Can you work these out from the model? Positions are in its coordinate system, mm. A direction names the side the tool comes from. Give positions to 0.01 mm unless a question says otherwise; leave off trailing zeros. Loops run counter-clockwise (first coordinate to the right, second up) from the corner with the lowest first, then second, coordinate; pieces in that order, holes last. Notation, with made-up numbers: (76.25, -26.5) - (103.25, -26.5) arc R22 cw to (103.25, -5.5) - close; hole circle Ø9 at (78, -14). An arc over 180 degrees is marked (long way). Answer in a Markdown table with one row per item.
from build123d import *

# Parameters (mm, degrees)
SKETCH_1_R      = 7.5
SKETCH_1_R_2    = 4
EXTRUDE_1_DEPTH = 24
SKETCH_4_W      = 1
SKETCH_4_H      = 1
FILLET_1_R      = 0.2


with BuildPart() as part:
    # 草图1 → 凸台-拉伸1 (new body)
    with BuildSketch(Plane.XY):
        Circle(SKETCH_1_R)
        Circle(SKETCH_1_R_2, mode=Mode.SUBTRACT)
    extrude(amount=EXTRUDE_1_DEPTH)

    # 草图4 → 切除-旋转1 (revolve, cut)
    with BuildSketch(Plane(origin=(0, 0, 0), x_dir=(0, 0, -1), z_dir=(1, 0, 0)), mode=Mode.PRIVATE) as cut_revolve_1_sk:
        with Locations((-20.5, 7.016772844)):
            Rectangle(SKETCH_4_W, SKETCH_4_H)
        with Locations((-3.5, 7.016772844)):
            Rectangle(SKETCH_4_W, SKETCH_4_H)
    revolve(cut_revolve_1_sk.sketch.rotate(Axis((0, 0, 0), (0, 0, 1)), 90), axis=Axis((0, 0, 0), (0, 0, 1)), mode=Mode.SUBTRACT)

    # 圆角1
    fillet_1_edges = [part.edges().sort_by_distance(p)[0] for p in [
        (-7.5, 0, 21),
        (-7.5, 0, 20),
        (-7.5, 0, 4),
        (-7.5, 0, 3),
    ]]
    fillet(fillet_1_edges, radius=FILLET_1_R)


solid = part.part
Q1. For pin 1 (5 mm diameter, centred on x = -5, z = 13, fed in from +Y); pin 2 (8 mm diameter, centred on y = 6, z = 8.5, fed in from +X); pin 3 (1.5 mm diameter, centred on x = -1, z = 6.5, fed in from -Y), each with a flat end and sliding along its axis, tell me the tip position at first contact or that it passes through.
Checked values:
| item | result |
|---|---|
| pin 1 | stops at y = 7.07 |
| pin 2 | stops at x = 7.23 |
| pin 3 | stops at y = -7.5 |
Q2. If we mould it in two halves opening along Z, with no side actions, what happens to faces 1 (the face through (1.413, 6.362, 20.493)), 2 (the face through (3, -3, 0)), 3 (the face through (-7.493, 0.33, 22.58))? For each: released by +Z, released by -Z, zero draft, split by the parting line, or undercut.
Checked values:
| item | result |
|---|---|
| face 1 | undercut |
| face 2 | released by -Z |
| face 3 | zero draft |
Q3. On a 3-axis mill with a long thin cutter (end or side, diameter ignored), from which of +Z, -Z, +X, -X, +Y, -Y can I reach the whole of each face in a straight line? I mean faces 4 (the face through (-3, -6, 3)), 5 (the face through (-7.493, 0.33, 1.38)). Say none if no direction works.
Checked values:
| item | result |
|---|---|
| face 4 | none |
| face 5 | +Z, -Z |
Q4. Imagine slicing it at C-C, the plane z = 8.75. Write out the boundary of the cut face in (x, y), and give its area (3 significant figures).
Checked values:
| item | result |
|---|---|
| outline | circle Ø15 at (0, 0); hole circle Ø8 at (0, 0) |
| area | 126 mm² |
Q5. If I drill on line 1 (Z direction, x = 5.75, y = -3.5); line 2 (Y direction, x = 0, z = 16.5); line 3 (Y direction, x = -2.75, z = 9.75), over which ranges is the centre line in solid material (lowest first)? Write a range as [from, to].
Checked values:
| item | result |
|---|---|
| line 1 | z = [0, 3], [4, 20], [21, 24] |
| line 2 | y = [-7.5, -4], [4, 7.5] |
| line 3 | y = [-6.98, -2.9], [2.9, 6.98] |
